from build123d import *

# Parameters (mm, degrees)
F0_R     = 17.75
F0_R_2   = 8.6
F1_DEPTH = 20
F2_R     = 19
F2_R_2   = 17.75
F3_DEPTH = 1.5
F4_SIZE  = 1
F5_SIZE  = 1


with BuildPart() as f1:
    # F0 (on Top) → F1 (new body)
    with BuildSketch(Plane.XY):
        Circle(F0_R)
        Circle(F0_R_2, mode=Mode.SUBTRACT)
    extrude(amount=F1_DEPTH)

    # F2 (on face) → F3 (join)
    with BuildSketch(Plane.XY.offset(20)):
        Circle(F2_R)
        Circle(F2_R_2, mode=Mode.SUBTRACT)
    extrude(amount=-F3_DEPTH)

    # F4
    f4_edges = [f1.edges().sort_by_distance(p)[0] for p in [
        (-17.75, 0, 0),
    ]]
    chamfer(f4_edges, length=F4_SIZE)

    # F5
    f5_edges = [f1.edges().sort_by_distance(p)[0] for p in [
        (-8.6, 0, 0),
    ]]
    chamfer(f5_edges, length=F5_SIZE)


solid = f1.part
Input: part model. Units: mm. Frame: model coordinates. Give positions to 0.01 mm unless a question says otherwise; leave off trailing zeros. Write each loop counter-clockwise with the first axis right and the second up, starting at its lowest first coordinate (ties: lowest second). Pieces come first, ordered by that corner, then holes. Notation, with made-up numbers: (0.5, 23.5) -> (29.5, 23.5) arc R17 ccw to (29.5, 48.5) -> close; hole circle Ø4 at (55.5, 33.5). An arc over 180 degrees is marked (long way). Use one line per item in the form item = value. Start each with the question number.
1) Section query A-A on y = 0. Return the cut outline in (x, z).
2) Ray query, probe 1 along Y at (x, z) = (0, 12.5); probe 2 along Z at (x, y) = (-16, 9); probe 3 along X at (y, z) = (-3, 5.5). Return the intervals inside material, ascending. Write a range as from..to.
3) Section query C-C on z = 3.75. Return the cut outline in (x, y), then the cut area to 3 significant figures.
4) Draft query along Y for faces 1 (the flat face through (-16, 9, 18.5)), 2 (the cylindrical face through (-8.59, 0.38, 10.37)), 3 (the cylindrical face through (-3.848, -17.328, 9.628)). Return one class per face: pulls with the +Y half, pulls with the -Y half, needs draft (parallel to the pull), parting line crosses it, or undercut.
5) Pin query (flat end, axial travel): pin 1 (10 mm diameter, centred on x = -0.5, z = 11.5, fed in from -Y); pin 2 (3 mm diameter, centred on y = -6.5, z = 4, fed in from +X); pin 3 (6 mm diameter, centred on x = -9, z = 16, fed in from +Y). Return the tip coordinate at first contact, or that it passes through.
Outcome:
q1.outline = (-19, 18.5) -> (-17.75, 18.5) -> (-17.75, 1) -> (-16.75, 0) -> (-9.6, 0) -> (-8.6, 1) -> (-8.6, 20) -> (-19, 20) -> close; (8.6, 1) -> (9.6, 0) -> (16.75, 0) -> (17.75, 1) -> (17.75, 18.5) -> (19, 18.5) -> (19, 20) -> (8.6, 20) -> close
q2.probe_1 = -17.75..-8.6, 8.6..17.75
q2.probe_2 = 18.5..20
q2.probe_3 = -17.49..-8.06, 8.06..17.49
q3.outline = circle Ø35.5 at (0, 0); hole circle Ø17.2 at (0, 0)
q3.area = 757 mm^2
q4.face_1 = needs draft
q4.face_2 = undercut
q4.face_3 = parting line crosses it
q5.pin_1 = -17.75
q5.pin_2 = 17.03
q5.pin_3 = 17.52
